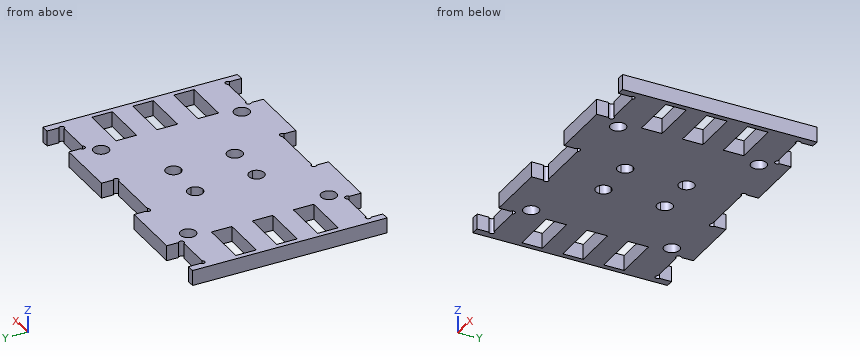
```python
from build123d import *

# Parameters (mm, degrees)
SKETCH_1_W          = 55
SKETCH_1_H          = 38
EXTRUDE_1_DEPTH     = 3
SKETCH_2_R          = 1.5
CUT_EXTRUDE_1_DEPTH = 30
SKETCH_3_W          = 8
SKETCH_3_H          = 3
CUT_EXTRUDE_2_DEPTH = 30
SKETCH_5_W          = 12
SKETCH_5_H          = 3
CUT_EXTRUDE_4_DEPTH = 10
SKETCH_6_W          = 9
SKETCH_6_H          = 4
CUT_EXTRUDE_5_DEPTH = 10
SKETCH_7_R          = 0.5
CUT_EXTRUDE_6_DEPTH = 10
CUT_EXTRUDE_7_DEPTH = 20


with BuildPart() as part:
    # 草图1 → 凸台-拉伸1 (new body)
    with BuildSketch(Plane.XY):
        Rectangle(SKETCH_1_W, SKETCH_1_H)
    extrude(amount=EXTRUDE_1_DEPTH)

    # 草图2 → 切除-拉伸1 (cut)
    with BuildSketch(Plane.XY.offset(3)):
        with Locations((16, 13.75)):
            Circle(SKETCH_2_R)
        with Locations((16, -13.75)):
            Circle(SKETCH_2_R)
        with Locations((-16, 13.75)):
            Circle(SKETCH_2_R)
        with Locations((-16, -13.75)):
            Circle(SKETCH_2_R)
    extrude(amount=-CUT_EXTRUDE_1_DEPTH, mode=Mode.SUBTRACT)

    # 草图3 → 切除-拉伸2 (cut)
    with BuildSketch(Plane.XY.offset(3)):
        with Locations((22, 17.5)):
            Rectangle(SKETCH_3_W, SKETCH_3_H)
        with Locations((22, -17.5)):
            Rectangle(SKETCH_3_W, SKETCH_3_H)
        with Locations((-22, 17.5)):
            Rectangle(SKETCH_3_W, SKETCH_3_H)
        with Locations((-22, -17.5)):
            Rectangle(SKETCH_3_W, SKETCH_3_H)
    extrude(amount=-CUT_EXTRUDE_2_DEPTH, mode=Mode.SUBTRACT)

    # 草图5 → 切除-拉伸4 (cut)
    with BuildSketch(Plane.XY.offset(3)):
        with Locations((0, -17.5)):
            Rectangle(SKETCH_5_W, SKETCH_5_H)
        with Locations((0, 17.5)):
            Rectangle(SKETCH_5_W, SKETCH_5_H)
    extrude(amount=-CUT_EXTRUDE_4_DEPTH, mode=Mode.SUBTRACT)

    # 草图6 → 切除-拉伸5 (cut)
    with BuildSketch(Plane(origin=(0, 0, 0), x_dir=(-1, 0, 0), z_dir=(0, 0, -1))):
        with Locations((-22, -8)):
            Rectangle(SKETCH_6_W, SKETCH_6_H)
        with Locations((-22, 0)):
            Rectangle(SKETCH_6_W, SKETCH_6_H)
        with Locations((-22, 8)):
            Rectangle(SKETCH_6_W, SKETCH_6_H)
        with Locations((22, -8)):
            Rectangle(SKETCH_6_W, SKETCH_6_H)
        with Locations((22, 0)):
            Rectangle(SKETCH_6_W, SKETCH_6_H)
        with Locations((22, 8)):
            Rectangle(SKETCH_6_W, SKETCH_6_H)
    extrude(amount=-CUT_EXTRUDE_5_DEPTH, mode=Mode.SUBTRACT)

    # 草图7 → 切除-拉伸6 (cut)
    with BuildSketch(Plane(origin=(0, 0, 0), x_dir=(-1, 0, 0), z_dir=(0, 0, -1))):
        with Locations((-18.212132034, -16.212132034)):
            Circle(SKETCH_7_R)
        with Locations((-25.787867966, -16.212132034)):
            Circle(SKETCH_7_R)
        with Locations((-25.787867966, 16.212132034)):
            Circle(SKETCH_7_R)
        with Locations((-18.212132034, 16.212132034)):
            Circle(SKETCH_7_R)
        with Locations((-5.787867966, -16.212132034)):
            Circle(SKETCH_7_R)
        with Locations((25.787867966, -16.212132034)):
            Circle(SKETCH_7_R)
        with Locations((18.212132034, -16.212132034)):
            Circle(SKETCH_7_R)
        with Locations((18.212132034, 16.212132034)):
            Circle(SKETCH_7_R)
        with Locations((25.787867966, 16.212132034)):
            Circle(SKETCH_7_R)
        with Locations((-5.787867966, 16.212132034)):
            Circle(SKETCH_7_R)
        with Locations((5.787867966, 16.212132034)):
            Circle(SKETCH_7_R)
        with Locations((5.787867966, -16.212132034)):
            Circle(SKETCH_7_R)
    extrude(amount=-CUT_EXTRUDE_6_DEPTH, mode=Mode.SUBTRACT)

    # 草图8 → 切除-拉伸7 (cut)
    with BuildSketch(Plane(origin=(0, 0, 0), x_dir=(-1, 0, 0), z_dir=(0, 0, -1))):
        with BuildLine():
            ThreePointArc((-2.5, 6), (-5.060660172, 7.060660172), (-4, 4.5))
            Line((-4, 4.5), (-4, 6))
            Line((-4, 6), (-2.5, 6))
        make_face()
        with BuildLine():
            Line((-4, 6), (-4, 4.5))
            ThreePointArc((-4, 4.5), (-2.939339828, 4.939339828), (-2.5, 6))
            Line((-2.5, 6), (-4, 6))
        make_face()
        with BuildLine():
            ThreePointArc((2.5, 6), (2.939339828, 4.939339828), (4, 4.5))
            Line((4, 4.5), (4, 6))
            Line((4, 6), (2.5, 6))
        make_face()
        with BuildLine():
            Line((4, 6), (4, 4.5))
            ThreePointArc((4, 4.5), (5.060660172, 4.939339828), (5.5, 6))
            ThreePointArc((5.5, 6), (4, 7.5), (2.5, 6))
            Line((2.5, 6), (4, 6))
        make_face()
        with BuildLine():
            ThreePointArc((5.5, -6), (5.060660172, -4.939339828), (4, -4.5))
            Line((4, -4.5), (4, -6))
            Line((4, -6), (2.5, -6))
            ThreePointArc((2.5, -6), (4, -7.5), (5.5, -6))
        make_face()
        with BuildLine():
            Line((4, -6), (4, -4.5))
            ThreePointArc((4, -4.5), (2.939339828, -4.939339828), (2.5, -6))
            Line((2.5, -6), (4, -6))
        make_face()
        with BuildLine():
            ThreePointArc((-2.5, -6), (-2.939339828, -4.939339828), (-4, -4.5))
            Line((-4, -4.5), (-4, -6))
            Line((-4, -6), (-2.5, -6))
        make_face()
        with BuildLine():
            Line((-4, -6), (-4, -4.5))
            ThreePointArc((-4, -4.5), (-5.060660172, -7.060660172), (-2.5, -6))
            Line((-2.5, -6), (-4, -6))
        make_face()
    extrude(amount=-CUT_EXTRUDE_7_DEPTH, mode=Mode.SUBTRACT)


solid = part.part
```
Can you work these out from the model? Positions are in its coordinate system, mm. Round coordinates to 2 decimals unless told otherwise and drop trailing zeros. Loops run counter-clockwise (first coordinate to the right, second up) from the corner with the lowest first, then second, coordinate; pieces in that order, holes last. Notation, with made-up numbers: M 42.5,36.5 L 64.5,36.5 A6 ccw 64.5,47.5 Z; hole C 12.5,21 d8. An arc over 180 degrees is marked long. Answer in a Markdown table with one row per item.
1. If we section it at D-D, the plane z = 2.2: Give the number of separate pieces and of enclosed holes in the cut face, plus the area to 3 significant figures.
Established:
| item | result |
|---|---|
| separate pieces | 1 |
| enclosed holes | 14 |
| area | 1,650 mm² |
2. If we section it at C-C, the plane x = -16: Please give me the cut outline in (y, z).
Established:
| item | result |
|---|---|
| outline | M -19,0 L -15.25,0 L -15.25,3 L -19,3 Z; M -12.25,0 L 12.25,0 L 12.25,3 L -12.25,3 Z; M 15.25,0 L 19,0 L 19,3 L 15.25,3 Z |
3. I'm going to push flat-ended pins straight in: pin 1 Ø1.5 at (x, y) = (-13.5, 3) entering from -Z; pin 2 Ø0.9 at (x, z) = (-22, 1.5) entering from +Y. Where does each tip first touch, or does it pass through?
Established:
| item | result |
|---|---|
| pin 1 | z = 0 |
| pin 2 | y = 16 |
4. If we section it at A-A, the plane x = 20: Please give me the cut outline in (y, z).
Established:
| item | result |
|---|---|
| outline | M -16,0 L -10,0 L -10,3 L -16,3 Z; M -6,0 L -2,0 L -2,3 L -6,3 Z; M 2,0 L 6,0 L 6,3 L 2,3 Z; M 10,0 L 16,0 L 16,3 L 10,3 Z |
5. If we section it at B-B, the plane y = -13.75: Please give me the cut outline in (x, z), plus the area to 3 significant figures.
Established:
| item | result |
|---|---|
| outline | M -27.5,0 L -17.5,0 L -17.5,3 L -27.5,3 Z; M -14.5,0 L 14.5,0 L 14.5,3 L -14.5,3 Z; M 17.5,0 L 27.5,0 L 27.5,3 L 17.5,3 Z |
| area | 147 mm² |
6. Please list where these lines run through material, in increasing order: line 1 (X direction, y = 1, z = 0.85); line 2 (Y direction, x = -21.5, z = 1.7); line 3 (Y direction, x = -4, z = 1.8). Write a range as from..to.
Established:
| item | result |
|---|---|
| line 1 | -27.5..-26.5, -17.5..17.5, 26.5..27.5 |
| line 2 | -16..-10, -6..-2, 2..6, 10..16 |
| line 3 | -16..-7.5, -4.5..4.5, 7.5..16 |
